```python
from build123d import *

# Parameters (mm, degrees)
F0_W     = 88.9
F0_H     = 101.6
F0_R     = 4.445
F0_R_2   = 2.5527
F1_DEPTH = 6.35
F2_W     = 88.9
F2_H     = 50.8
F3_DEPTH = 6.35
F4_R     = 4.96062
F5_DEPTH = 25.4
F6_SIZE  = 3.048


with BuildPart() as f1:
    # F0 (on Top) → F1 (new body)
    with BuildSketch(Plane.XY):
        Rectangle(F0_W, F0_H)
        with Locations((-38.1, 6.35)):
            Circle(F0_R, mode=Mode.SUBTRACT)
        with Locations((-19.05, 6.35)):
            Circle(F0_R_2, mode=Mode.SUBTRACT)
        with Locations((-38.1, 44.45)):
            Circle(F0_R, mode=Mode.SUBTRACT)
        with Locations((-19.05, 44.45)):
            Circle(F0_R_2, mode=Mode.SUBTRACT)
        with Locations((0, 6.35)):
            Circle(F0_R, mode=Mode.SUBTRACT)
        with Locations((19.05, 6.35)):
            Circle(F0_R_2, mode=Mode.SUBTRACT)
        with Locations((38.1, 6.35)):
            Circle(F0_R, mode=Mode.SUBTRACT)
        with Locations((0, 44.45)):
            Circle(F0_R, mode=Mode.SUBTRACT)
        with Locations((19.05, 44.45)):
            Circle(F0_R_2, mode=Mode.SUBTRACT)
        with Locations((38.1, 44.45)):
            Circle(F0_R, mode=Mode.SUBTRACT)
    extrude(amount=F1_DEPTH)

    # F2 (on face) → F3 (join)
    with BuildSketch(Plane.XY.offset(6.35)):
        with Locations((0, -25.4)):
            Rectangle(F2_W, F2_H)
    extrude(amount=F3_DEPTH)

    # F4 (on face) → F5 (cut)
    with BuildSketch(Plane.XY.offset(12.7)):
        with Locations((-19.05, -38.1)):
            Circle(F4_R)
        with Locations((19.05, -38.1)):
            Circle(F4_R)
    extrude(amount=-F5_DEPTH, mode=Mode.SUBTRACT)

    # F6
    f6_edges = [f1.edges().sort_by_distance(p)[0] for p in [
        (-21.6027, 44.45, 6.35),
        (16.4973, 44.45, 6.35),
        (16.4973, 6.35, 6.35),
        (-21.6027, 6.35, 6.35),
    ]]
    chamfer(f6_edges, length=F6_SIZE)


solid = f1.part
```
Could you check a few things on this model? Use its own coordinates, in mm. A direction names the side the tool comes from. Round coordinates to 2 decimals unless told otherwise and drop trailing zeros. Write each loop counter-clockwise with the first axis right and the second up, starting at its lowest first coordinate (ties: lowest second). Pieces come first, ordered by that corner, then holes. Notation, with made-up numbers: M 21,-2.5 L 45,-2.5 A24 cw 45,14.5 Z; hole C 13.5,-36 d8. An arc over 180 degrees is marked long. Write each question's results on one line, items separated by ' | '. Start each with the question number.
1. Thinking about a two-plate mould opening in X: for faces 3 (the face through (16.35, 6.47, 3.45)), 4 (the face through (-44.45, -12, 5)), 5 (the face through (-1, 1, 0)), which applies, +X half, -X half, draft (parallel to the pull), parting line (faces both ways), or undercut?
2. I'm going to push flat-ended pins straight in: pin 1 Ø6.5 at (x, y) = (-19.05, 44.45) entering from +Z; pin 2 Ø6 at (x, y) = (19.05, 6.35) entering from +Z; pin 3 Ø10 at (x, y) = (32.5, 29.5) entering from +Z. Where does each tip first touch, or does it pass through?
3. Imagine slicing it at C-C on y = -38.1. List the corners of the cut face in (x, z) for me, and give its area (3 significant figures).
4. I need wall thicknesses on L1, parallel to Y at x = 0, z = 2.5 (3 decimals); L2, parallel to Y at x = -19.05, z = 1.3; L3, parallel to Y at x = -19.05, z = 6.75. Which ranges of each line are inside material? Lowest first, please. Write a range as from..to.
5. Imagine slicing it at A-A on y = 44.45. List the corners of the cut face in (x, z) for me (3 decimals), and give its area (3 significant figures).
6. On a 3-axis mill with a long thin cutter (end or side, diameter ignored), from which of +Z, -Z, +X, -X, +Y, -Y can I reach the whole of each face in a straight line? I mean faces 1 (the face through (-1, 0, 9)), 2 (the face through (-0.579, 48.857, 3.131)). Say none if no direction works.
7. Imagine slicing it at B-B on x = -38.1. List the corners of the cut face in (y, z) for me (3 decimals).
8. Imagine slicing it at D-D on x = -19.05. List the corners of the cut face in (y, z) for me, and give its area (3 significant figures).
Result sheet:
1) face 3: undercut | face 4: -X half | face 5: draft
2) pin 1: stops at z = 4 | pin 2: stops at z = 3.75 | pin 3: stops at z = 6.35
3) outline: M -44.45,0 L -24.01,0 L -24.01,12.7 L -44.45,12.7 Z; M -14.09,0 L 14.09,0 L 14.09,12.7 L -14.09,12.7 Z; M 24.01,0 L 44.45,0 L 44.45,12.7 L 24.01,12.7 Z | area: 877 mm^2
4) L1: y = -50.8..1.905, 10.795..40.005, 48.895..50.8 | L2: y = -50.8..-43.06, -33.14..3.8, 8.9..41.9, 47..50.8 | L3: y = -50.8..-43.06, -33.14..0
5) outline: M -44.45,0 L -42.545,0 L -42.545,6.35 L -44.45,6.35 Z; M -33.655,0 L -21.603,0 L -21.603,3.302 L -24.651,6.35 L -33.655,6.35 Z; M -16.497,0 L -4.445,0 L -4.445,6.35 L -13.449,6.35 L -16.497,3.302 Z; M 4.445,0 L 16.497,0 L 16.497,3.302 L 13.449,6.35 L 4.445,6.35 Z; M 21.603,0 L 33.655,0 L 33.655,6.35 L 24.651,6.35 L 21.603,3.302 Z; M 42.545,0 L 44.45,0 L 44.45,6.35 L 42.545,6.35 Z | area: 312 mm^2
6) face 1: +Z, +X, -X, +Y | face 2: +Z, -Z
7) outline: M -50.8,0 L 1.905,0 L 1.905,6.35 L 0,6.35 L 0,12.7 L -50.8,12.7 Z; M 10.795,0 L 40.005,0 L 40.005,6.35 L 10.795,6.35 Z; M 48.895,0 L 50.8,0 L 50.8,6.35 L 48.895,6.35 Z
8) outline: M -50.8,0 L -43.06,0 L -43.06,12.7 L -50.8,12.7 Z; M -33.14,0 L 3.8,0 L 3.8,3.3 L 0.75,6.35 L 0,6.35 L 0,12.7 L -33.14,12.7 Z; M 8.9,0 L 41.9,0 L 41.9,3.3 L 38.85,6.35 L 11.95,6.35 L 8.9,3.3 Z; M 47,0 L 50.8,0 L 50.8,6.35 L 50.05,6.35 L 47,3.3 Z | area: 758 mm^2
